Answer from the drawing. Dimensions are ordinates in mm from the lowest x, y and z of the part. A direction names the side the tool comes from. Round coordinates to 2 decimals unless told otherwise and drop trailing zeros. Write each loop counter-clockwise with the first axis right and the second up, starting at its lowest first coordinate (ties: lowest second). Pieces come first, ordered by that corner, then holes.
1. Find section D-D (x = 2). Write down the section's boundary in (y, z) (1 decimal), and give its area (3 significant figures).
2. Find section A-A (x = 11.5). Write down the section's boundary in (y, z) (1 decimal).
3. A tool of negligible diameter and unlimited length cuts with its end or side. For the marked faces 1 and 2, from which of +Z, -Z, +X, -X, +Y, -Y can it reach the whole face along a straight path? Write none if from no direction.
4. Flat-ended cylindrical pins translate along their axes: pin 1 Ø6 at (x, z) = (4, 10) entering from -Y; pin 2 Ø14.5 at (x, y) = (15, 28.5) entering from -Z; pin 3 Ø4 at (x, y) = (13.5, 5) entering from -Z. Find the tip coordinate at first contact, or state that the pin passes through.
5. Find section B-B (y = 13). Write down the section's boundary in (x, z) (1 decimal).
6. Straight lines are drawn through the part: probe 1 along X at (y, z) = (8, 76) (1 decimal); probe 2 along X at (y, z) = (12, 77.75) (1 decimal); probe 3 along Z at (x, y) = (11.5, 21.5). For each, find the intervals that lie inside material, in ascending order.
7. Find section C-C (z = 26.5). Write down the section's boundary in (x, y) (1 decimal).
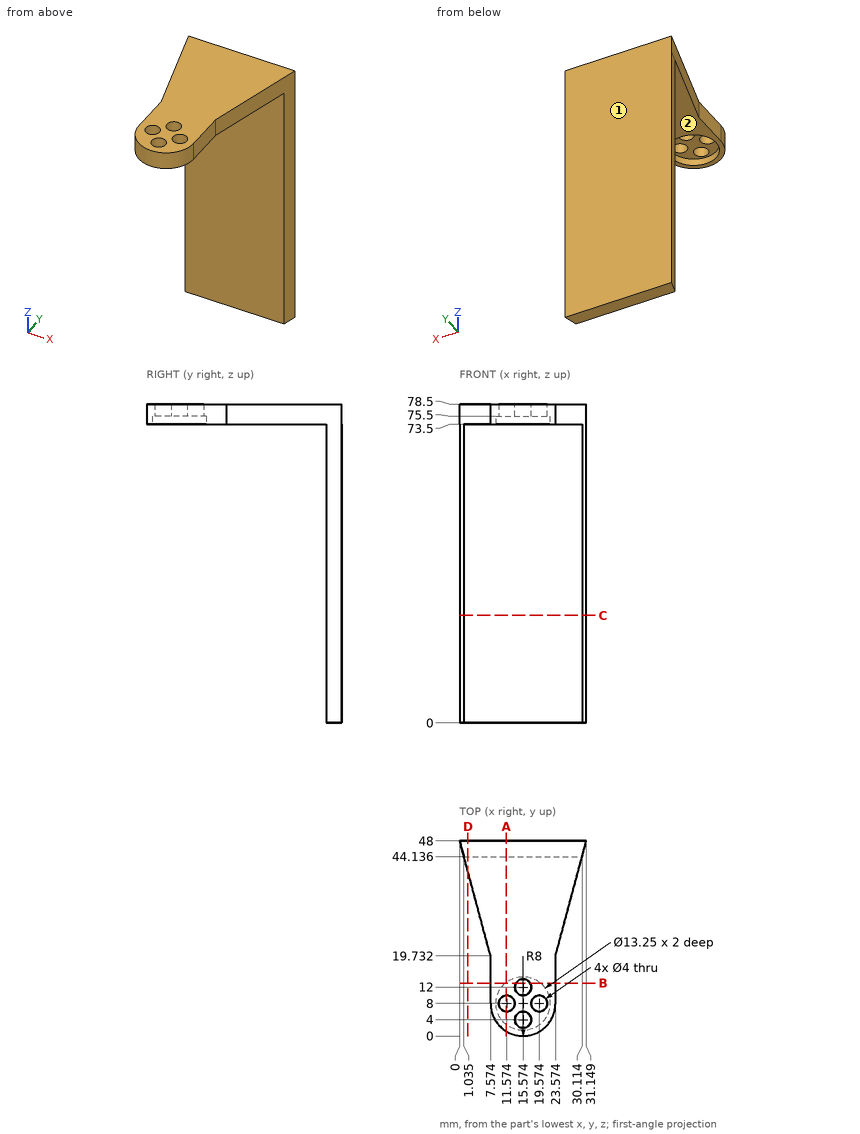
Worked answers:
1. outline: (40.5, 73.5) - (44.1, 73.5) - (44.1, 0) - (48, 0) - (48, 78.5) - (40.5, 78.5) - close
1. area: 321 mm2
2. outline: (1.1, 73.5) - (2.8, 73.5) - (2.8, 75.5) - (6, 75.5) - (6, 78.5) - (1.1, 78.5) - close; (10, 75.5) - (13.2, 75.5) - (13.2, 73.5) - (44.1, 73.5) - (44.1, 0) - (48, 0) - (48, 78.5) - (10, 78.5) - close
3. face 1: +Z, -Z, +X, -X, +Y
3. face 2: -Z, +X, -X, -Y
4. pin 1: stops at y = 44.14
4. pin 2: stops at z = 73.5
4. pin 3: stops at z = 75.5
5. outline: (7.6, 73.5) - (11.2, 73.5) - (11.2, 75.5) - (13.8, 75.5) - (13.8, 78.5) - (7.6, 78.5) - close; (17.3, 75.5) - (19.9, 75.5) - (19.9, 73.5) - (23.6, 73.5) - (23.6, 78.5) - (17.3, 78.5) - close
6. probe 1: x = 7.6 to 9.6, 13.6 to 17.6, 21.6 to 23.6
6. probe 2: x = 7.6 to 13.6, 17.6 to 23.6
6. probe 3: z = 73.5 to 78.5
7. outline: (0, 48) - (1, 44.1) - (30.1, 44.1) - (31.1, 48) - close
